Geometry check sheet. Reference: drawing and pictorial views, mm from the part's lowest x, y, z. A direction names the side the tool comes from. Round coordinates to 2 decimals unless told otherwise and drop trailing zeros. Order: outer loops, then holes, each group sorted by start corner. A loop starts at its lowest first (then second) coordinate and runs counter-clockwise, first axis right, second up. Notation, with made-up numbers: (-31, -32) -> (0, -32) arc R25 ccw to (0, -11) -> close; hole circle Ø6 at (-15.75, -25). An arc over 180 degrees is marked (long way). Put each result on its own line as item: value.
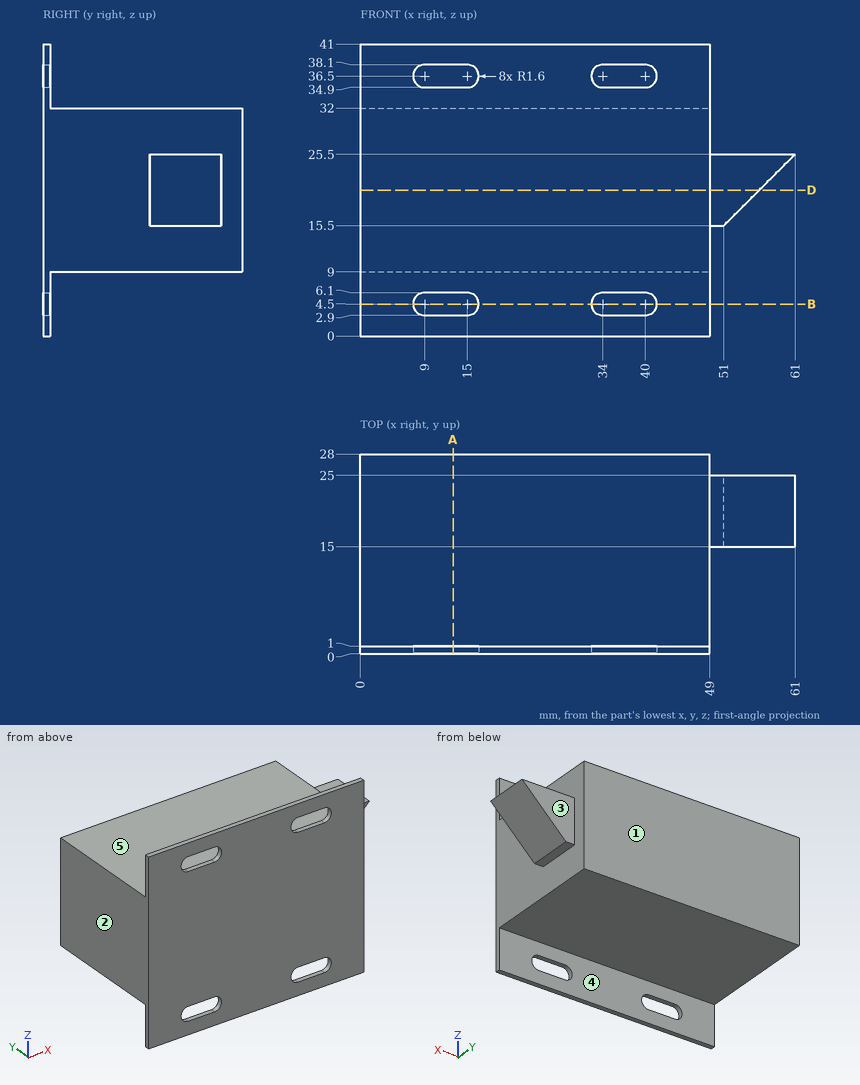
Item 1: Material ranges on line 1 along X through (y, z) = (5, 29.5); line 2 along Z through (x, y) = (37, 23); line 3 along Y through (x, z) = (15.5, 7.5), recorded low to high.
Geometry check:
line 1: 0 to 49
line 2: 9 to 32
line 3: 0 to 1
Item 2: Sectioned sample at D-D, the plane z = 20.5. Record the boundary of the cut face in (x, y).
Geometry check:
outline: (0, 0) -> (49, 0) -> (49, 15) -> (56, 15) -> (56, 25) -> (49, 25) -> (49, 28) -> (0, 28) -> close
Item 3: Depth check by flat-ended pin: pin 1 Ø5 at (y, z) = (8.5, 32.5) entering from +X; pin 2 Ø8 at (x, z) = (56, 22.5) entering from +Y; pin 3 Ø5 at (x, z) = (54.5, 20) entering from -Y. Enter the tip coordinate at first touch or a pass-through.
Geometry check:
pin 1: x = 49
pin 2: y = 25
pin 3: y = 15
Item 4: Sectioned sample at B-B, the plane z = 4.5. Record the boundary of the cut face in (x, y).
Geometry check:
outline: (0, 0) -> (7.4, 0) -> (7.4, 1) -> (0, 1) -> close; (16.6, 0) -> (32.4, 0) -> (32.4, 1) -> (16.6, 1) -> close; (41.6, 0) -> (49, 0) -> (49, 1) -> (41.6, 1) -> close
Item 5: Tool access check on the marked faces 1, 2, 3, 4 and 5. Record the directions out of +Z, -Z, +X, -X, +Y, -Y that give a thin tool (end or side, any length) a straight path to the whole face; none if there is none.
Geometry check:
face 1: +Z, -Z, +X, -X, +Y
face 2: +Z, -Z, -X, +Y, -Y
face 3: +Z, -Z, +X, +Y
face 4: -Z, +X, -X, +Y
face 5: +Z, +X, -X, +Y
Item 6: Sectioned sample at A-A, the plane x = 13. Record the boundary of the cut face in (y, z), then the cut area to 3 significant figures.
Geometry check:
outline: (0, 0) -> (1, 0) -> (1, 2.9) -> (0, 2.9) -> close; (0, 6.1) -> (1, 6.1) -> (1, 9) -> (28, 9) -> (28, 32) -> (1, 32) -> (1, 34.9) -> (0, 34.9) -> close; (0, 38.1) -> (1, 38.1) -> (1, 41) -> (0, 41) -> close
area: 656 mm2
